Can you work these out from the model? Positions are in its coordinate system, mm. Face numbers are marked on the shaded views. A direction names the side the tool comes from. Coordinates: 2 decimals unless noted, no trailing zeros. Order: outer loops, then holes, each group sorted by start corner. A loop starts at its lowest first (then second) coordinate and runs counter-clockwise, first axis right, second up. Notation, with made-up numbers: (62, 27.25) -> (101, 27.25) arc R16 cw to (101, 35.25) -> close; hole circle Ø8 at (28.5, 1). An arc over 180 degrees is marked (long way). Write item = value, one per line.
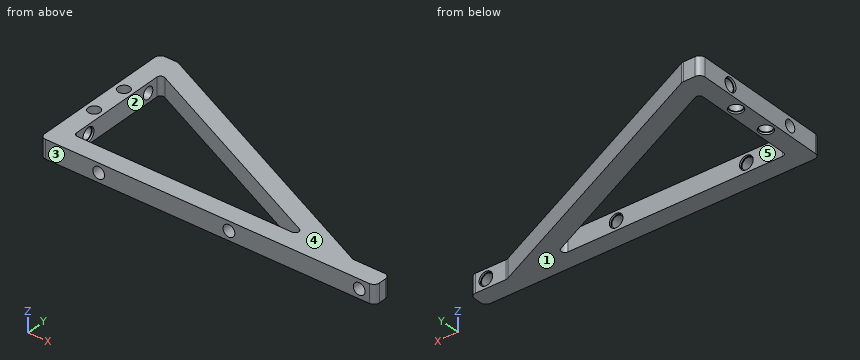
```python
from build123d import *

# Parameters (mm, degrees)
ESQUISSE1_W                         = 180
ESQUISSE1_H                         = 80
BOSS_EXTRU_1_DEPTH                  = 10
ESQUISSE2_W                         = 170
ESQUISSE2_H                         = 70
ENL_V_MAT_EXTRU_1_DEPTH             = 1
ENL_V_MAT_EXTRU_1_DEPTH_BACK        = 11
BOSS_EXTRU_2_DEPTH                  = 10
ENL_V_MAT_EXTRU_2_REACH             = 82
ESQUISSE4_R                         = 3.15
ENL_V_MAT_EXTRU_2_DIRECTION_2_DEPTH = 1
ESQUISSE5_R                         = 3.65
ENL_V_MAT_EXTRU_3_DEPTH             = 1
ENL_V_MAT_EXTRU_4_REACH             = 182
ESQUISSE6_R                         = 3.15
ENL_V_MAT_EXTRU_4_DIRECTION_2_DEPTH = 1
ESQUISSE7_R                         = 3.65
ENL_V_MAT_EXTRU_5_DEPTH             = 1
ESQUISSE8_R                         = 3.65
ENL_V_MAT_EXTRU_6_DEPTH             = 1
CONG_1_R                            = 2
CONG_2_R                            = 3
ESQUISSE9_R                         = 3.15
ENL_V_MAT_EXTRU_7_DEPTH             = 1
ENL_V_MAT_EXTRU_7_DEPTH_BACK        = 11
ENL_V_START                         = -10
ESQUISSE10_R                        = 3.65
ENL_V_MAT_EXTRU_8_DEPTH             = 1


with BuildPart() as part:
    # Esquisse1 → Boss.-Extru.1 (new body)
    with BuildSketch(Plane.XY):
        with Locations((90, 40)):
            Rectangle(ESQUISSE1_W, ESQUISSE1_H)
    extrude(amount=BOSS_EXTRU_1_DEPTH)

    # Esquisse2 → Enlèv. mat.-Extru.1 (cut, two sides)
    with BuildSketch(Plane.XY.offset(10)) as enl_v_mat_extru_1_sk:
        with Locations((95, 45)):
            Rectangle(ESQUISSE2_W, ESQUISSE2_H)
    extrude(amount=ENL_V_MAT_EXTRU_1_DEPTH, mode=Mode.SUBTRACT)
    extrude(enl_v_mat_extru_1_sk.sketch, amount=-ENL_V_MAT_EXTRU_1_DEPTH_BACK, mode=Mode.SUBTRACT)

    # Esquisse3 → Boss.-Extru.2 (add)
    with BuildSketch(Plane.XY.offset(10)):
        Polygon((10, 80), (160.115484436, 10), (136.453468604, 10), (10, 68.96622081), align=None)
    extrude(amount=-BOSS_EXTRU_2_DEPTH)

    # Esquisse4 → Enlèv. mat.-Extru.2 (cut, up to next)
    with BuildSketch(Plane.XZ, mode=Mode.PRIVATE) as enl_v_mat_extru_2_sk1:
        with Locations((101.5, 5)):
            Circle(ESQUISSE4_R)
    enl_v_mat_extru_2_tool1 = extrude(enl_v_mat_extru_2_sk1.sketch, amount=-ENL_V_MAT_EXTRU_2_REACH, mode=Mode.PRIVATE) & part.part
    add(enl_v_mat_extru_2_tool1.solids().sort_by_distance((101.5, 0, 5))[0], mode=Mode.SUBTRACT)
    # Esquisse4 → Enlèv. mat.-Extru.2 (cut, up to next)
    with BuildSketch(Plane.XZ, mode=Mode.PRIVATE) as enl_v_mat_extru_2_sk2:
        with Locations((171.5, 5)):
            Circle(ESQUISSE4_R)
    enl_v_mat_extru_2_tool2 = extrude(enl_v_mat_extru_2_sk2.sketch, amount=-ENL_V_MAT_EXTRU_2_REACH, mode=Mode.PRIVATE) & part.part
    add(enl_v_mat_extru_2_tool2.solids().sort_by_distance((171.5, 0, 5))[0], mode=Mode.SUBTRACT)
    # Esquisse4 → Enlèv. mat.-Extru.2 (cut, up to next)
    with BuildSketch(Plane.XZ, mode=Mode.PRIVATE) as enl_v_mat_extru_2_sk3:
        with Locations((31.5, 5)):
            Circle(ESQUISSE4_R)
    enl_v_mat_extru_2_tool3 = extrude(enl_v_mat_extru_2_sk3.sketch, amount=-ENL_V_MAT_EXTRU_2_REACH, mode=Mode.PRIVATE) & part.part
    add(enl_v_mat_extru_2_tool3.solids().sort_by_distance((31.5, 0, 5))[0], mode=Mode.SUBTRACT)

    # Esquisse4 → Enlèv. mat.-Extru.2 direction 2 (cut)
    with BuildSketch(Plane.XZ):
        with Locations((101.5, 5)):
            Circle(ESQUISSE4_R)
        with Locations((171.5, 5)):
            Circle(ESQUISSE4_R)
        with Locations((31.5, 5)):
            Circle(ESQUISSE4_R)
    extrude(amount=ENL_V_MAT_EXTRU_2_DIRECTION_2_DEPTH, mode=Mode.SUBTRACT)

    # Esquisse5 → Enlèv. mat.-Extru.3 (cut)
    with BuildSketch(Plane(origin=(0, 10, 0), x_dir=(1, 0, 0), z_dir=(0, 1, 0))):
        with Locations((101.5, -5)):
            Circle(ESQUISSE5_R)
        with Locations((171.5, -5)):
            Circle(ESQUISSE5_R)
        with Locations((31.5, -5)):
            Circle(ESQUISSE5_R)
    extrude(amount=-ENL_V_MAT_EXTRU_3_DEPTH, mode=Mode.SUBTRACT)

    # Esquisse6 → Enlèv. mat.-Extru.4 (cut, up to next)
    with BuildSketch(Plane.ZY, mode=Mode.PRIVATE) as enl_v_mat_extru_4_sk1:
        with Locations((5, 60)):
            Circle(ESQUISSE6_R)
    enl_v_mat_extru_4_tool1 = extrude(enl_v_mat_extru_4_sk1.sketch, amount=-ENL_V_MAT_EXTRU_4_REACH, mode=Mode.PRIVATE) & part.part
    add(enl_v_mat_extru_4_tool1.solids().sort_by_distance((0, 60, 5))[0], mode=Mode.SUBTRACT)
    # Esquisse6 → Enlèv. mat.-Extru.4 (cut, up to next)
    with BuildSketch(Plane.ZY, mode=Mode.PRIVATE) as enl_v_mat_extru_4_sk2:
        with Locations((5, 20)):
            Circle(ESQUISSE6_R)
    enl_v_mat_extru_4_tool2 = extrude(enl_v_mat_extru_4_sk2.sketch, amount=-ENL_V_MAT_EXTRU_4_REACH, mode=Mode.PRIVATE) & part.part
    add(enl_v_mat_extru_4_tool2.solids().sort_by_distance((0, 20, 5))[0], mode=Mode.SUBTRACT)

    # Esquisse6 → Enlèv. mat.-Extru.4 direction 2 (cut)
    with BuildSketch(Plane.ZY):
        with Locations((5, 60)):
            Circle(ESQUISSE6_R)
        with Locations((5, 20)):
            Circle(ESQUISSE6_R)
    extrude(amount=ENL_V_MAT_EXTRU_4_DIRECTION_2_DEPTH, mode=Mode.SUBTRACT)

    # Esquisse7 → Enlèv. mat.-Extru.5 (cut)
    with BuildSketch(Plane.ZY):
        with Locations((5, 60)):
            Circle(ESQUISSE7_R)
    extrude(amount=-ENL_V_MAT_EXTRU_5_DEPTH, mode=Mode.SUBTRACT)

    # Esquisse8 → Enlèv. mat.-Extru.6 (cut)
    with BuildSketch(Plane(origin=(10, 0, 0), x_dir=(0, 0, -1), z_dir=(1, 0, 0))):
        with Locations((-5, 20)):
            Circle(ESQUISSE8_R)
    extrude(amount=-ENL_V_MAT_EXTRU_6_DEPTH, mode=Mode.SUBTRACT)

    # Congé1
    cong_1_edges = [part.edges().sort_by_distance(p)[0] for p in [
        (10, 10, 5),
        (10, 68.96622081, 5),
        (136.453468604, 10, 5),
    ]]
    fillet(cong_1_edges, radius=CONG_1_R)

    # Congé2
    cong_2_edges = [part.edges().sort_by_distance(p)[0] for p in [
        (10, 80, 5),
        (180, 10, 5),
        (160.115484436, 10, 5),
        (0, 80, 5),
        (180, 0, 5),
        (0, 0, 5),
    ]]
    fillet(cong_2_edges, radius=CONG_2_R)

    # Esquisse9 → Enlèv. mat.-Extru.7 (cut, two sides)
    with BuildSketch(Plane.XY.offset(10)) as enl_v_mat_extru_7_sk:
        with Locations((5, 50)):
            Circle(ESQUISSE9_R)
        with Locations((5, 30)):
            Circle(ESQUISSE9_R)
    extrude(amount=ENL_V_MAT_EXTRU_7_DEPTH, mode=Mode.SUBTRACT)
    extrude(enl_v_mat_extru_7_sk.sketch, amount=-ENL_V_MAT_EXTRU_7_DEPTH_BACK, mode=Mode.SUBTRACT)

    # Esquisse10 → Enlèv. mat.-Extru.8 (cut)
    with BuildSketch(Plane.XY.offset(10).offset(ENL_V_START)):
        with Locations((5, 50)):
            Circle(ESQUISSE10_R)
        with Locations((5, 30)):
            Circle(ESQUISSE10_R)
    extrude(amount=ENL_V_MAT_EXTRU_8_DEPTH, mode=Mode.SUBTRACT)


solid = part.part
```
Item 1: If we mould it in two halves opening along Y, with no side actions, what happens to the marked faces 3, 4 and 5? For each: pulls with the +Y half, pulls with the -Y half, needs draft (parallel to the pull), parting line crosses it, or undercut.
A:
face_3 = pulls with the -Y half
face_4 = needs draft
face_5 = undercut
Item 2: For the marked faces 1 and 2, which set-ups out of +Z, -Z, +X, -X, +Y, -Y let a thin tool reach every point of the face, with its end or its side?
A:
face_1 = -Z, +X, -X, +Y, -Y
face_2 = +Z, -Z
Item 3: I want a section at C-C, the plane x = 31.5. Please give me the cut outline in (y, z).
A:
outline = (0, 0) -> (10, 0) -> (10, 1.35) -> (9, 1.35) -> (9, 1.85) -> (0, 1.85) -> close; (0, 8.15) -> (9, 8.15) -> (9, 8.65) -> (10, 8.65) -> (10, 10) -> (0, 10) -> close; (58.94, 0) -> (69.97, 0) -> (69.97, 10) -> (58.94, 10) -> close
Item 4: I want a section at A-A, the plane x = 171.5. Please give me the cut outline in (y, z).
A:
outline = (0, 0) -> (10, 0) -> (10, 1.35) -> (9, 1.35) -> (9, 1.85) -> (0, 1.85) -> close; (0, 8.15) -> (9, 8.15) -> (9, 8.65) -> (10, 8.65) -> (10, 10) -> (0, 10) -> close
Item 5: I want a section at D-D, the plane y = 20. Please give me the cut outline in (x, z), plus the area to 3 significant figures.
A:
outline = (0, 0) -> (10, 0) -> (10, 1.35) -> (9, 1.35) -> (9, 1.85) -> (0, 1.85) -> close; (0, 8.15) -> (9, 8.15) -> (9, 8.65) -> (10, 8.65) -> (10, 10) -> (0, 10) -> close; (115.01, 0) -> (138.67, 0) -> (138.67, 10) -> (115.01, 10) -> close
area = 273 mm2
Item 6: I'm going to push flat-ended pins straight in: P1, Ø4, axis at x = 18.5, z = 8, coming from the +Y side; P2, Ø2, axis at y = 20.5, z = 4.5, coming from the +X side; P3, Ø3.5, axis at x = 4, y = 50.5, coming from the -Z side; P4, Ø5.5, axis at y = 20, z = 5, coming from the +X side. Where does each tip first touch, or does it pass through?
A:
P1 = 76.97
P2 = 139.74
P3 = through
P4 = 144.57
Item 7: I want a section at B-B, the plane z = 5. Give the number of separate pieces and of enclosed holes in the cut face, plus the area to 3 significant figures.
A:
separate_pieces = 5
enclosed_holes = 2
area = 3,650 mm2
Item 8: If I drill on probe 1 along Y at (x, z) = (5, 0.45); probe 2 along Z at (x, y) = (101.5, 9.75); probe 3 along Y at (x, z) = (0.5, 5), over which ranges is the centre line in solid material (lowest first)?
A:
probe_1 = 0 to 26.35, 33.65 to 46.35, 53.65 to 80
probe_2 = 0 to 1.35, 8.65 to 10
probe_3 = 1.34 to 16.85, 23.15 to 56.35, 63.65 to 78.66
